```python
from build123d import *

# Parameters (mm, degrees)
PAD001_DEPTH    = 2.55
SKETCH_R        = 1.175
POCKET_DEPTH    = 0.301
PAD_DEPTH       = 0.3
POCKET001_DEPTH = 3.851
SKETCH004_W     = 0.3
SKETCH004_H     = 7.5
PAD002_DEPTH    = 3.3
FILLET_R        = 0.5
SKETCH005_W     = 11.05
SKETCH005_H     = 0.3
PAD003_DEPTH    = 3.55
PAD004_DEPTH    = 3.1
PAD005_DEPTH    = 0.3


with BuildPart() as part:
    # Sketch001 (on YZ_Plane of Origin) → Pad001 (new body, symmetric)
    with BuildSketch(Plane.YZ):
        with BuildLine():
            Line((15.25, 0), (10.75, 0))
            ThreePointArc((10.25, 0.5), (10.396447, 0.146447), (10.75, 0))
            Line((10.25, 0.5), (10.25, 3.05))
            ThreePointArc((10.25, 3.05), (10.103553, 3.403553), (9.75, 3.55))
            Line((9.75, 3.55), (-9.75, 3.55))
            ThreePointArc((-9.75, 3.55), (-10.103553, 3.403553), (-10.25, 3.05))
            Line((-10.25, 3.05), (-10.25, 0.5))
            ThreePointArc((-10.75, 0), (-10.396447, 0.146447), (-10.25, 0.5))
            Line((-10.75, 0), (-15.25, 0))
            Line((-15.25, 0), (-15.25, 0.3))
            Line((-15.25, 0.3), (-11.05, 0.3))
            ThreePointArc((-11.05, 0.3), (-10.696447, 0.446447), (-10.55, 0.8))
            Line((-10.55, 0.8), (-10.55, 3.85))
            Line((10.55, 3.85), (-10.55, 3.85))
            Line((10.55, 0.8), (10.55, 3.85))
            ThreePointArc((10.55, 0.8), (10.696447, 0.446447), (11.05, 0.3))
            Line((15.25, 0.3), (11.05, 0.3))
            Line((15.25, 0), (15.25, 0.3))
        make_face()
    extrude(amount=PAD001_DEPTH, both=True)

    # Sketch (on Face18 of Pad001) → Pocket (cut, through all)
    with BuildSketch(Plane.XY.offset(0.3)):
        with Locations((0, 12.95)):
            Circle(SKETCH_R)
        with Locations((0, -12.95)):
            Circle(SKETCH_R)
    extrude(amount=-POCKET_DEPTH, mode=Mode.SUBTRACT)

    # Sketch002 → Pad (join)
    with BuildSketch(Plane.XY.offset(3.85)):
        with BuildLine():
            Line((-5.75, 10.55), (-10.5, 3.75))
            Line((-10.5, 3.75), (-10.5, -3.75))
            Line((-5.75, -10.55), (-10.5, -3.75))
            Line((-5.75, -10.55), (6.3, -10.55))
            ThreePointArc((6.3, -10.55), (9.107984, -8.606042), (8.2769, -5.293484))
            ThreePointArc((8.2769, 5.293484), (6.09, 0), (8.2769, -5.293484))
            ThreePointArc((8.2769, 5.293484), (9.107984, 8.606042), (6.3, 10.55))
            Line((-5.75, 10.55), (6.3, 10.55))
        make_face()
    extrude(amount=-PAD_DEPTH)

    # Sketch003 (on Face30 of Pad) → Pocket001 (cut, through all)
    with BuildSketch(Plane.XY.offset(3.85)):
        with BuildLine():
            ThreePointArc((0.134679, 7.1), (-5.65, 5.55), (0.134679, 4))
            Line((5.35, 4), (0.134679, 4))
            Line((5.35, 7.1), (5.35, 4))
            Line((0.134679, 7.1), (5.35, 7.1))
        make_face()
        with BuildLine():
            ThreePointArc((0.134679, -4), (-5.65, -5.55), (0.134679, -7.1))
            Line((0.134679, -7.1), (5.35, -7.1))
            Line((5.35, -7.1), (5.35, -4))
            Line((5.35, -4), (0.134679, -4))
        make_face()
    extrude(amount=-POCKET001_DEPTH, mode=Mode.SUBTRACT)

    # Sketch004 (on Face11 of Pocket001) → Pad002 (join)
    with BuildSketch(Plane(origin=(0, 0, 3.55), x_dir=(1, 0, 0), z_dir=(0, 0, -1))):
        with Locations((-10.35, 0)):
            Rectangle(SKETCH004_W, SKETCH004_H)
    extrude(amount=PAD002_DEPTH)

    # Fillet
    fillet_edges = [part.edges().sort_by_distance(p)[0] for p in [
        (-10.2, 0, 3.55),
    ]]
    fillet(fillet_edges, radius=FILLET_R)

    # Sketch005 (on Face11 of Pocket001) → Pad003 (join)
    with BuildSketch(Plane(origin=(0, 0, 3.55), x_dir=(1, 0, 0), z_dir=(0, 0, -1))):
        with Locations((-0.225, 10.4)):
            Rectangle(SKETCH005_W, SKETCH005_H)
        with Locations((-0.225, -10.4)):
            Rectangle(SKETCH005_W, SKETCH005_H)
    extrude(amount=PAD003_DEPTH)

    # Sketch006 (on XZ_Plane of Origin) → Pad004 (join)
    with BuildSketch(Plane.XZ.offset(4)):
        Polygon((-0.85, 1.35), (5.35, 3.85), (5.35, 3.55), (-0.85, 1.05), align=None)
    pad004 = extrude(amount=PAD004_DEPTH)

    # Mirrored: Pad004 across XZ
    add(pad004.mirror(Plane.XZ))

    # Sketch007 (on XY_Plane of Origin) → Pad005 (join)
    with BuildSketch(Plane.XY.offset(1.05)):
        with BuildLine():
            Line((-0.85, 4), (-1.75, 4))
            ThreePointArc((-1.75, 4), (-3.3, 5.55), (-1.75, 7.1))
            Line((-1.75, 7.1), (-0.85, 7.1))
            Line((-0.85, 7.1), (-0.85, 4))
        make_face()
    pad005 = extrude(amount=PAD005_DEPTH)

    # Mirrored001: Pad005 across Sketch007 H_Axis
    add(pad005.mirror(Plane(origin=(0, 0, 1.05), x_dir=(0, 0, 1), z_dir=(0, 1, 0))))


solid = part.part
```
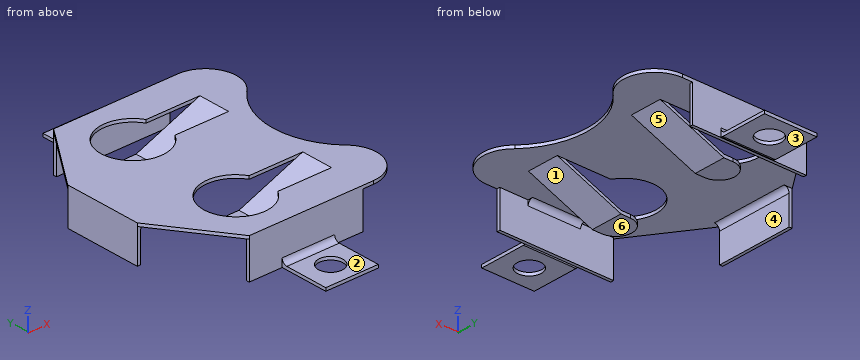
Model file for the job. Use its own axes, mm. Face numbers are marked on the shaded views. A direction names the side the tool comes from. Coordinates: 2 decimals unless noted, no trailing zeros. Loops run counter-clockwise (first coordinate to the right, second up) from the corner with the lowest first, then second, coordinate; pieces in that order, holes last. Notation, with made-up numbers: (80.25, 80.25) -> (116.25, 80.25) arc R31 cw to (116.25, 119.25) -> close; hole circle Ø1 at (42, -16.75). An arc over 180 degrees is marked (long way). Answer as a JSON object with one key per item and string values.
Q1. Cut at B-B (x = 4). List the corners of the cut face in (y, z).
Report:
{"outline": "(-10.55, 0) -> (-10.25, 0) -> (-10.25, 3.55) -> (-7.1, 3.55) -> (-7.1, 3.85) -> (-10.55, 3.85) -> close; (-7.1, 3.01) -> (-4, 3.01) -> (-4, 3.31) -> (-7.1, 3.31) -> close; (-4, 3.55) -> (4, 3.55) -> (4, 3.85) -> (-4, 3.85) -> close; (4, 3.01) -> (7.1, 3.01) -> (7.1, 3.31) -> (4, 3.31) -> close; (7.1, 3.55) -> (10.25, 3.55) -> (10.25, 0) -> (10.55, 0) -> (10.55, 3.85) -> (7.1, 3.85) -> close"}
Q2. Flat gauge pins, fed straight in: P1, Ø1.2, axis at x = 0.5, z = 1.5, coming from the -Y side; P2, Ø0.6, axis at x = -10, z = 2.5, coming from the -Y side; P3, Ø0.6, axis at x = -10.5, z = 2.5, coming from the +Y side. Where does each tip first touch, or does it go through?
Report:
{"P1": "stops at y = -10.55", "P2": "stops at y = -3.75", "P3": "stops at y = 3.75"}
Q3. Pull direction Y, two halves, no side cores. Call the marked faces 1 and 2: released by +Y, released by -Y, zero draft, split by the parting line, or undercut.
Report:
{"face 1": "undercut", "face 2": "zero draft"}
Q4. Cut at D-D (x = -4). List the corners of the cut face in (y, z), and give its area (3 significant figures).
Report:
{"outline": "(-10.55, 0) -> (-10.25, 0) -> (-10.25, 3.55) -> (-8.29, 3.55) -> (-8.29, 3.85) -> (-10.55, 3.85) -> close; (-2.81, 3.55) -> (2.81, 3.55) -> (2.81, 3.85) -> (-2.81, 3.85) -> close; (8.29, 3.55) -> (10.25, 3.55) -> (10.25, 0) -> (10.55, 0) -> (10.55, 3.85) -> (8.29, 3.85) -> close", "area": "5.17 mm2"}
Q5. Cut at C-C (z = 1.65). List the corners of the cut face in (x, y), and give its area (3 significant figures).
Report:
{"outline": "(-10.5, -3.75) -> (-10.2, -3.75) -> (-10.2, 3.75) -> (-10.5, 3.75) -> close; (-5.75, -10.55) -> (5.3, -10.55) -> (5.3, -10.25) -> (-5.75, -10.25) -> close; (-5.75, 10.25) -> (5.3, 10.25) -> (5.3, 10.55) -> (-5.75, 10.55) -> close; (-0.11, -7.1) -> (0.64, -7.1) -> (0.64, -4) -> (-0.11, -4) -> close; (-0.11, 4) -> (0.64, 4) -> (0.64, 7.1) -> (-0.11, 7.1) -> close", "area": "13.5 mm2"}
Q6. 3-axis set-ups, long thin cutter, end or side, ignore diameter. For the marked faces 3, 4, 5 and 6: which of +Z, -Z, +X, -X, +Y, -Y reach the whole face in a straight line?
Report:
{"face 3": "-Z, +X, -X, +Y, -Y", "face 4": "-Z, +X, +Y, -Y", "face 5": "-Z, +X", "face 6": "-Z, +X, -X"}
Q7. Cut at A-A (y = -12.95). List the corners of the cut face in (x, z) (3 decimals).
Report:
{"outline": "(-2.55, 0) -> (-1.175, 0) -> (-1.175, 0.3) -> (-2.55, 0.3) -> close; (1.175, 0) -> (2.55, 0) -> (2.55, 0.3) -> (1.175, 0.3) -> close"}
Q8. Probe probe 1 along Y at (x, z) = (0, 0.2) (3 decimals); probe 2 along Y at (x, z) = (2, 1.25); probe 3 along Z at (x, y) = (0, -3). List the from-to ranges inside material, lowest first.
Report:
{"probe 1": "y = -15.25 to -14.125, -11.775 to -10.25, 10.25 to 11.775, 14.125 to 15.25", "probe 2": "y = -10.55 to -10.25, 10.25 to 10.55", "probe 3": "z = 3.55 to 3.85"}
